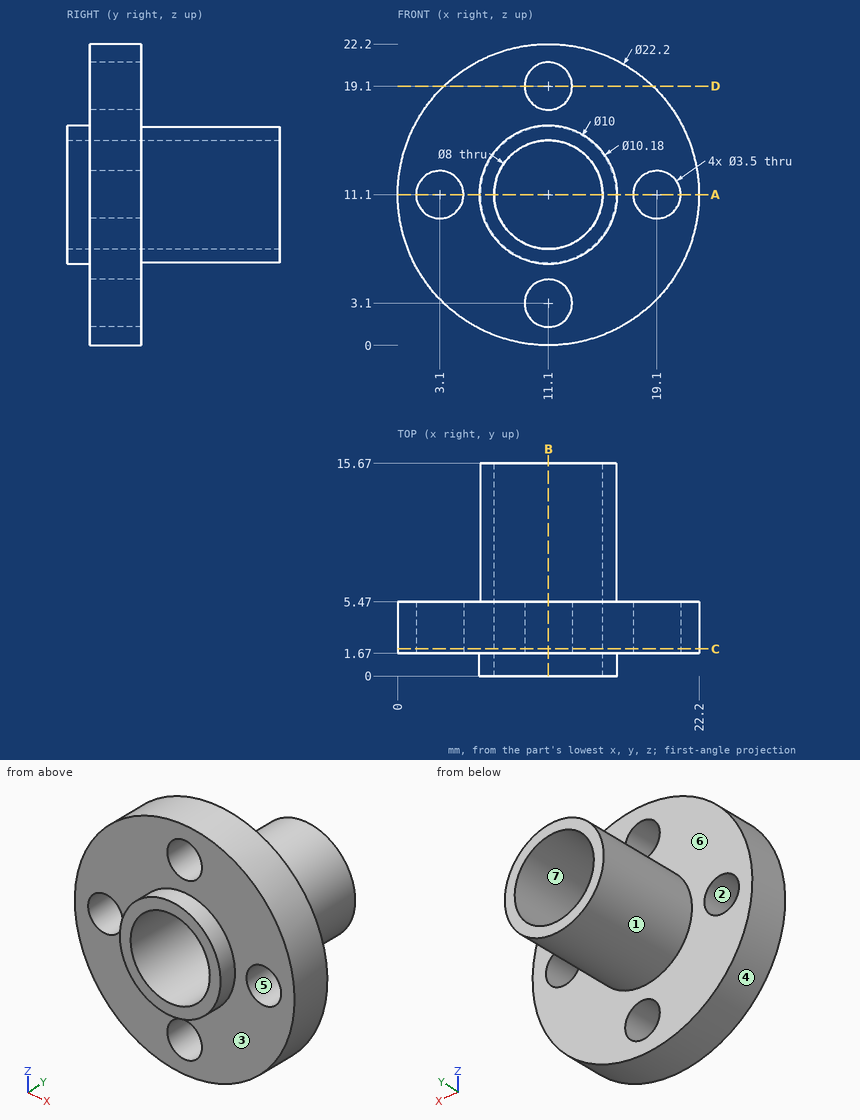
Here's the drawing with two shaded views (mm, measured from the low corner). I have some questions. A direction names the side the tool comes from. Give positions to 0.01 mm unless a question says otherwise; leave off trailing zeros. Write each loop counter-clockwise with the first axis right and the second up, starting at its lowest first coordinate (ties: lowest second). Pieces come first, ordered by that corner, then holes. Notation, with made-up numbers: (9.5, 75.5) -> (31.5, 75.5) arc R32 ccw to (31.5, 103.5) -> close; hole circle Ø2 at (28, 18). An arc over 180 degrees is marked (long way). One line per item, written item: value.
Q1. Imagine slicing it at B-B on x = 11.1. Please give me the cut outline in (y, z), and give its area (3 significant figures).
Results found:
outline: (0, 6.01) -> (1.67, 6.01) -> (1.67, 4.85) -> (5.47, 4.85) -> (5.47, 6.1) -> (15.67, 6.1) -> (15.67, 7.1) -> (0, 7.1) -> close; (0, 15.1) -> (15.67, 15.1) -> (15.67, 16.1) -> (5.47, 16.1) -> (5.47, 17.35) -> (1.67, 17.35) -> (1.67, 16.19) -> (0, 16.19) -> close; (1.67, 0) -> (5.47, 0) -> (5.47, 1.35) -> (1.67, 1.35) -> close; (1.67, 20.85) -> (5.47, 20.85) -> (5.47, 22.2) -> (1.67, 22.2) -> close
area: 51.4 mm^2
Q2. Imagine slicing it at C-C on y = 2. Please give me the cut outline in (x, z).
Results found:
outline: circle Ø22.2 at (11.1, 11.1); hole circle Ø3.5 at (3.1, 11.1); hole circle Ø8 at (11.1, 11.1); hole circle Ø3.5 at (11.1, 3.1); hole circle Ø3.5 at (11.1, 19.1); hole circle Ø3.5 at (19.1, 11.1)
Q3. For P1, Ø4, axis at y = 11.5, z = 5, coming from the -X side; P2, Ø4, axis at y = 7.5, z = 10, coming from the -X side; P3, Ø1, axis at x = 10, z = 20, coming from the +Y side, each with a flat end and sliding along its axis, tell me the tip position at first contact or that it passes through.
Results found:
P1: stops at x = 8.24
P2: stops at x = 6.1
P3: stops at y = 5.47
Q4. Which directions (+Z, -Z, +X, -X, +Y, -Y) give clear straight access to the entire face, cutting with the end or side of a thin tool? Please do the marked faces 1, 2 and 3.
Results found:
face 1: +Y
face 2: +Y, -Y
face 3: -Y
Q5. Please list where these lines run through material, in increasing order: line 1 (X direction, y = 4.5, z = 11.1); line 2 (Z direction, x = 12.5, y = 5.25). Write a range as [from, to].
Results found:
line 1: x = [0, 1.35], [4.85, 7.1], [15.1, 17.35], [20.85, 22.2]
line 2: z = [0.09, 2.05], [4.15, 7.35], [14.85, 18.05], [20.15, 22.11]
Q6. Imagine slicing it at A-A on z = 11.1. Please give me the cut outline in (x, y).
Results found:
outline: (0, 1.67) -> (1.35, 1.67) -> (1.35, 5.47) -> (0, 5.47) -> close; (4.85, 1.67) -> (6.01, 1.67) -> (6.01, 0) -> (7.1, 0) -> (7.1, 15.67) -> (6.1, 15.67) -> (6.1, 5.47) -> (4.85, 5.47) -> close; (15.1, 0) -> (16.19, 0) -> (16.19, 1.67) -> (17.35, 1.67) -> (17.35, 5.47) -> (16.1, 5.47) -> (16.1, 15.67) -> (15.1, 15.67) -> close; (20.85, 1.67) -> (22.2, 1.67) -> (22.2, 5.47) -> (20.85, 5.47) -> close
Q7. Imagine slicing it at D-D on z = 19.1. Please give me the cut outline in (x, y), and give its area (3 significant figures).
Results found:
outline: (3.41, 1.67) -> (9.35, 1.67) -> (9.35, 5.47) -> (3.41, 5.47) -> close; (12.85, 1.67) -> (18.79, 1.67) -> (18.79, 5.47) -> (12.85, 5.47) -> close
area: 45.2 mm^2
Q8. We'd pull the mould along Z, two halves only. Please class the marked faces 4, 5, 6 and 7: +Z half, -Z half, draft (parallel to the pull), parting line (faces both ways), or undercut.
Results found:
face 4: parting line
face 5: undercut
face 6: draft
face 7: undercut
